Could you check a few things on this drawing? It's one solid part, dimensions in mm from its lowest x, y, z. A direction names the side the tool comes from. Give positions to 0.01 mm unless a question says otherwise; leave off trailing zeros. Order: outer loops, then holes, each group sorted by start corner. A loop starts at its lowest first (then second) coordinate and runs counter-clockwise, first axis right, second up.
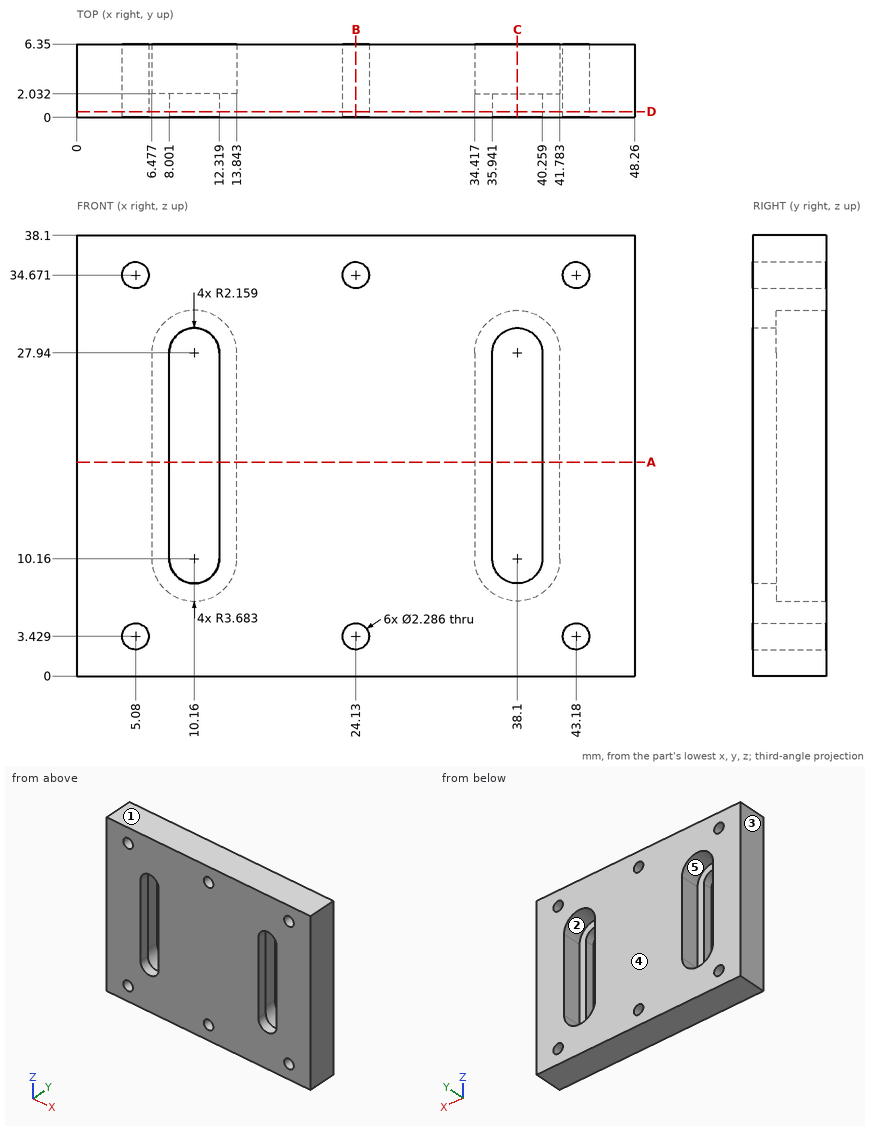
1) Suppose I cut it at C-C (x = 38.1). Please give me the cut outline in (y, z).
2) Suppose I cut it at B-B (x = 24.13). Please give me the cut outline in (y, z), and give its area (3 significant figures).
3) Suppose I cut it at A-A (z = 18.5). Please give me the cut outline in (x, y), and give its area (3 significant figures).
4) Suppose I cut it at D-D (y = 0.5). Give the number of separate pieces and of enclosed holes in the cut face, and give its area (3 significant figures).
5) If I drill on line 1 (X direction, y = 2.5, z = 23.5); line 2 (X direction, y = 0.5, z = 20); line 3 (Z direction, x = 5.08, y = 4), over which ranges is the centre line in solid material (lowest first)?
6) I'm going to push flat-ended pins straight in: pin 1 Ø4 at (x, z) = (37.5, 11.5) entering from +Y; pin 2 Ø1.8 at (x, z) = (43.18, 34.671) entering from -Y. Where does each tip first touch, or does it pass through?
7) Which directions (+Z, -Z, +X, -X, +Y, -Y) give clear straight access to the entire face, cutting with the end or side of a thin tool? Please do the marked faces 4 and 5.
8) We'd pull the mould along X, two halves only. Please class the marked faces 1, 2 and 3: +X half, -X half, draft (parallel to the pull), parting line (faces both ways), or undercut.
Results:
1. outline: (0, 0) - (6.35, 0) - (6.35, 6.48) - (2.03, 6.48) - (2.03, 8) - (0, 8) - close; (0, 30.1) - (2.03, 30.1) - (2.03, 31.62) - (6.35, 31.62) - (6.35, 38.1) - (0, 38.1) - close
2. outline: (0, 0) - (6.35, 0) - (6.35, 2.29) - (0, 2.29) - close; (0, 4.57) - (6.35, 4.57) - (6.35, 33.53) - (0, 33.53) - close; (0, 35.81) - (6.35, 35.81) - (6.35, 38.1) - (0, 38.1) - close
2. area: 213 mm2
3. outline: (0, 0) - (8, 0) - (8, 2.03) - (6.48, 2.03) - (6.48, 6.35) - (0, 6.35) - close; (12.32, 0) - (35.94, 0) - (35.94, 2.03) - (34.42, 2.03) - (34.42, 6.35) - (13.84, 6.35) - (13.84, 2.03) - (12.32, 2.03) - close; (40.26, 0) - (48.26, 0) - (48.26, 6.35) - (41.78, 6.35) - (41.78, 2.03) - (40.26, 2.03) - close
3. area: 225 mm2
4. separate pieces: 1
4. enclosed holes: 8
4. area: 1,630 mm2
5. line 1: x = 0 to 6.48, 13.84 to 34.42, 41.78 to 48.26
5. line 2: x = 0 to 8, 12.32 to 35.94, 40.26 to 48.26
5. line 3: z = 0 to 2.29, 4.57 to 33.53, 35.81 to 38.1
6. pin 1: stops at y = 2.03
6. pin 2: passes through
7. face 4: +Z, -Z, +X, -X, +Y
7. face 5: +Y
8. face 1: draft
8. face 2: undercut
8. face 3: -X half
